Input: part model. Units: mm. Frame: model coordinates. A direction names the side the tool comes from. Round coordinates to 2 decimals unless told otherwise and drop trailing zeros. Loops run counter-clockwise (first coordinate to the right, second up) from the corner with the lowest first, then second, coordinate; pieces in that order, holes last.
(1) First-contact query: pin 1 Ø1.3 at (x, z) = (-120, 2.5) entering from +Y; pin 2 Ø3 at (y, z) = (-178.5, 3) entering from +X. Flat tips, straight axial feed; report the tip coordinate or a pass-through.
(2) Cut plane A-A, the plane y = -216.5. Output: boundary loops of the cut face in (x, z), and give its area (4 significant figures).
(3) Access query for faces 1 (the face through (-121, -166.255, 2)), 2 (the face through (-103, -194.97, 2)), 3 (the face through (-121.35, -176, 2)), 4 (the face through (-199, -252.972, 2)). Directions: +Z, -Z, +X, -X, +Y, -Y. A direction counts if a zero-diameter tool reaches every point of the face in a straight line with its end or side. Return the directions, or none.
(4) Draft query along X for faces 5 (the face through (-216.716, -168.867, 2.465)), 6 (the face through (-42, -252.972, 2)), 7 (the face through (-126.498, -223, 2)), 8 (the face through (-148.498, -223, 2)). Return one class per face: released by +X, released by -X, zero draft, split by the parting line, or undercut.
(5) Cut plane C-C, the plane z = 3.4. Give the number of separate pieces and of enclosed holes in the cut face, and give its area (3 significant figures).
(6) Cut plane B-B, the plane x = -107. Output: boundary loops of the cut face in (y, z), and give its area (3 significant figures).
(7) Line query: line 1 (X direction, y = -205, z = 4.5); line 2 (Y direction, x = -75.5, z = 0.9); line 3 (X direction, y = -178.5, z = 2.05). Output: solid intervals per line, ascending.
from build123d import *

# Parameters (mm, degrees)
SKETCH1_R           = 1.9
SKETCH1_R_2         = 2.15
SKETCH1_W           = 2.7
SKETCH1_H           = 10
BOSS_EXTRUDE1_DEPTH = 5
BOSS_EXTRUDE2_DEPTH = 5
SKETCH2_2_W         = 42
SKETCH2_2_H         = 22
CUT_EXTRUDE1_DEPTH  = 5


with BuildPart() as part:
    # Sketch1 → Boss-Extrude1 (new body)
    with BuildSketch(Plane.XY):
        with BuildLine():
            Line((-243.5, -252.972288794), (-152.498180394, -252.972288794))
            ThreePointArc((-152.498180394, -252.972288794), (-149.669753269, -251.800715919), (-148.498180394, -248.972288794))
            Line((-148.498180394, -248.972288794), (-148.498180394, -196.970492539))
            ThreePointArc((-148.498180394, -196.970492539), (-147.912393957, -195.556278976), (-146.498180394, -194.970492539))
            Line((-146.498180394, -194.970492539), (-128.498180394, -194.970492539))
            ThreePointArc((-128.498180394, -194.970492539), (-127.083966832, -195.556278976), (-126.498180394, -196.970492539))
            Line((-126.498180394, -196.970492539), (-126.498180394, -248.972288794))
            ThreePointArc((-126.498180394, -248.972288794), (-125.326607519, -251.800715919), (-122.498180394, -252.972288794))
            Line((-122.498180394, -252.972288794), (-117.377838381, -252.972288794))
            ThreePointArc((-117.377838381, -252.972288794), (-114.549411256, -251.800715919), (-113.377838381, -248.972288794))
            Line((-113.377838381, -248.972288794), (-113.377838381, -196.970492539))
            ThreePointArc((-113.377838381, -196.970492539), (-112.792051943, -195.556278976), (-111.377838381, -194.970492539))
            Line((-111.377838381, -194.970492539), (-93.377838381, -194.970492539))
            ThreePointArc((-93.377838381, -194.970492539), (-91.963624819, -195.556278976), (-91.377838381, -196.970492539))
            Line((-91.377838381, -196.970492539), (-91.377838381, -248.972288794))
            ThreePointArc((-91.377838381, -248.972288794), (-90.206265506, -251.800715919), (-87.377838381, -252.972288794))
            Line((-87.377838381, -252.972288794), (5.5, -252.972288794))
            ThreePointArc((5.5, -252.972288794), (8.328427125, -251.800715919), (9.5, -248.972288794))
            Line((9.5, -248.972288794), (9.5, -187.432851256))
            add(Edge.make_bspline(
                [(-75.569581097, -152.972288794), (-30.278898356, -163.497720658), (9.5, -187.432851256)],
                knots=[0, 0, 0, 1, 1, 1], degree=2))
            Line((-75.569581097, -152.972288794), (-118.65, -152.972288794))
            Line((-118.65, -152.972288794), (-118.65, -162.972288794))
            Line((-118.65, -162.972288794), (-121.35, -162.972288794))
            Line((-121.35, -162.972288794), (-121.35, -152.972288794))
            Line((-121.35, -152.972288794), (-164.430418903, -152.972288794))
            add(Edge.make_bspline(
                [(-164.430418903, -152.972288794), (-207.794171984, -154.134737544), (-247.5, -171.407059989)],
                knots=[0, 0, 0, 1, 1, 1], degree=2))
            Line((-247.5, -171.407059989), (-247.5, -248.972288794))
            ThreePointArc((-247.5, -248.972288794), (-246.328427125, -251.800715919), (-243.5, -252.972288794))
        make_face()
        with Locations((0, -192.921490239)):
            Circle(SKETCH1_R, mode=Mode.SUBTRACT)
        with Locations((0, -242.921490239)):
            Circle(SKETCH1_R, mode=Mode.SUBTRACT)
        with Locations(Location((-237.993794987, -242.921490239, 0), (0, 0, 180))):
            Circle(SKETCH1_R, mode=Mode.SUBTRACT)
        with Locations(Location((-237.993794987, -194.970492539, 0), (0, 0, 180))):
            Circle(SKETCH1_R, mode=Mode.SUBTRACT)
        with Locations((-166.815366628, -192.921490239)):
            Circle(SKETCH1_R_2, mode=Mode.SUBTRACT)
        with Locations((-166.815366628, -242.921490239)):
            Circle(SKETCH1_R_2, mode=Mode.SUBTRACT)
        with Locations((-75.569581097, -192.921490239)):
            Circle(SKETCH1_R_2, mode=Mode.SUBTRACT)
        with Locations((-75.569581097, -242.921490239)):
            Circle(SKETCH1_R_2, mode=Mode.SUBTRACT)
        with Locations((-120, -176.407059989)):
            Rectangle(SKETCH1_W, SKETCH1_H, mode=Mode.SUBTRACT)
    extrude(amount=BOSS_EXTRUDE1_DEPTH)

    # Sketch2 → Boss-Extrude2 (add)
    with BuildSketch(Plane(origin=(0, 0, 0), x_dir=(-1, 0, 0), z_dir=(0, 0, -1))):
        with BuildLine():
            Line((247.500000017, -171.407059996), (185.05842867, -166.255233236))
            Line((185.05842867, -166.255233236), (54.943181018, -166.255233236))
            Line((54.943181018, -166.255233236), (34.928242723, -165.547963122))
            add(Edge.make_bspline(
                [(58.315946636, -155.801157817), (45.893296778, -158.75444176), (34.928242723, -165.547963122)],
                knots=[0, 0, 0, 1, 1, 1], degree=2))
            add(Edge.make_bspline(
                [(58.315946636, -155.801157817), (63.424678897, -156.071648314), (70.654281497, -151.741484529)],
                knots=[0, 0, 0, 0.409142446, 0.409142446, 0.409142446], degree=2))
            add(Edge.make_bspline(
                [(113.326199409, -148.857198457), (91.886453079, -148.664892877), (70.654281497, -151.741484529)],
                knots=[0, 0, 0, 1, 1, 1], degree=2))
            Line((113.326199409, -148.857198457), (126.673800592, -148.857198457))
            add(Edge.make_bspline(
                [(185.597069482, -153.384908978), (156.563126475, -146.928393886), (126.673800592, -148.857198457)],
                knots=[0, 0, 0, 1, 1, 1], degree=2))
            add(Edge.make_bspline(
                [(185.597069482, -153.384908978), (219.13818523, -148.75209862), (247.500000017, -171.407059996)],
                knots=[0, 0, 0, 1, 1, 1], degree=2))
        make_face()
    extrude(amount=-BOSS_EXTRUDE2_DEPTH)

    # Sketch2_2 → Cut-Extrude1 (cut)
    with BuildSketch(Plane(origin=(0, 0, 0), x_dir=(-1, 0, 0), z_dir=(0, 0, -1))):
        with BuildLine():
            Line((247.500000017, -171.407059996), (185.05842867, -166.255233236))
            Line((185.05842867, -166.255233236), (54.943181018, -166.255233236))
            Line((54.943181018, -166.255233236), (34.928242723, -165.547963122))
            add(Edge.make_bspline(
                [(58.315946636, -155.801157817), (45.893296778, -158.75444176), (34.928242723, -165.547963122)],
                knots=[0, 0, 0, 1, 1, 1], degree=2))
            add(Edge.make_bspline(
                [(58.315946636, -155.801157817), (63.424678897, -156.071648314), (70.654281497, -151.741484529)],
                knots=[0, 0, 0, 0.409142446, 0.409142446, 0.409142446], degree=2))
            add(Edge.make_bspline(
                [(113.326199409, -148.857198457), (91.886453079, -148.664892877), (70.654281497, -151.741484529)],
                knots=[0, 0, 0, 1, 1, 1], degree=2))
            Line((113.326199409, -148.857198457), (126.673800592, -148.857198457))
            add(Edge.make_bspline(
                [(185.597069482, -153.384908978), (156.563126475, -146.928393886), (126.673800592, -148.857198457)],
                knots=[0, 0, 0, 1, 1, 1], degree=2))
            add(Edge.make_bspline(
                [(185.597069482, -153.384908978), (219.13818523, -148.75209862), (247.500000017, -171.407059996)],
                knots=[0, 0, 0, 1, 1, 1], degree=2))
        make_face()
        with Locations((131.194571019, -151.63222762)):
            Rectangle(SKETCH2_2_W, SKETCH2_2_H)
    extrude(amount=-CUT_EXTRUDE1_DEPTH, mode=Mode.SUBTRACT)


solid = part.part
Reported:
1. pin 1: stops at y = -166.26
1. pin 2: stops at x = -3.59
2. outline: (-247.5, 0) - (-148.5, 0) - (-148.5, 5) - (-247.5, 5) - close; (-126.5, 0) - (-113.38, 0) - (-113.38, 5) - (-126.5, 5) - close; (-91.38, 0) - (9.5, 0) - (9.5, 5) - (-91.38, 5) - close
2. area: 1,065 mm2
3. face 1: +Z, -Z, -X, +Y
3. face 2: +Z, -Z, -Y
3. face 3: +Z, -Z
3. face 4: +Z, -Z, +X, -X, -Y
4. face 5: released by -X
4. face 6: zero draft
4. face 7: undercut
4. face 8: undercut
5. separate pieces: 1
5. enclosed holes: 9
5. area: 19,000 mm2
6. outline: (-194.97, 0) - (-166.26, 0) - (-166.26, 5) - (-194.97, 5) - close
6. area: 144 mm2
7. line 1: x = -247.5 to -148.5, -126.5 to -113.38, -91.38 to 9.5
7. line 2: y = -252.97 to -245.07, -240.77 to -195.07, -190.77 to -166.26
7. line 3: x = -247.5 to -121.35, -118.65 to -6.43
